Can you work these out from the model? Positions are in its coordinate system, mm. Face numbers are marked on the shaded views. A direction names the side the tool comes from. Give positions to 0.01 mm unless a question says otherwise; leave off trailing zeros. Loops run counter-clockwise (first coordinate to the right, second up) from the corner with the lowest first, then second, coordinate; pieces in that order, holes last. Notation, with made-up numbers: (-14.75, -28.5) - (5.25, -28.5) arc R35 ccw to (5.25, 10.5) - close; hole circle Ø5 at (7, 29.5). An arc over 180 degrees is marked (long way). Answer as a JSON object with one key per item and string values. Group by question number.
Item 1: Which directions (+Z, -Z, +X, -X, +Y, -Y) give clear straight access to the entire face, cutting with the end or side of a thin tool? Please do the marked faces 1, 2 and 3.
Item 2: Thinking about a two-plate mould opening in Y: for the marked faces 4, 5 and 6, which applies, pulls with the +Y half, pulls with the -Y half, needs draft (parallel to the pull), parting line crosses it, or undercut?
Item 3: Please list where these lines run through material, in increasing order: L1, parallel to Y at x = 4, z = 6; L2, parallel to X at y = 6.5, z = 9.75; L3, parallel to Z at x = -2.75, y = -3.5.
Item 4: Will these pins go through, and if not, where does the flat tip stop? pin 1 (1.5 mm diameter, centred on x = -0.5, y = -4.5, fed in from -Z); pin 2 (4.5 mm diameter, centred on x = 0.5, z = 4, fed in from -Y).
Item 5: Suppose I cut it at C-C on x = 0.25. Write out the boundary of the cut face in (y, z).
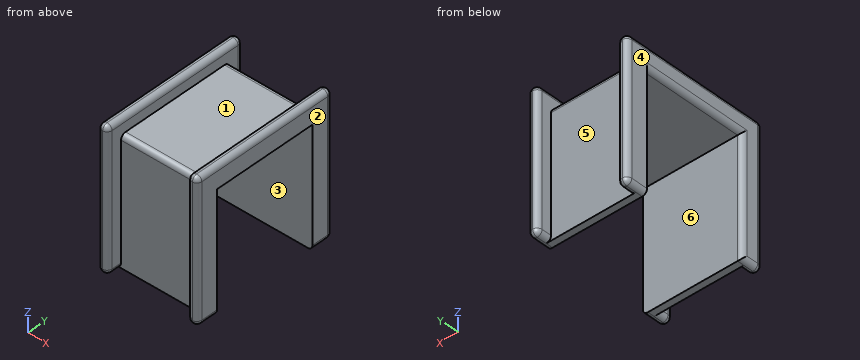
from build123d import *

# Parameters (mm, degrees)
F0_W     = 10.16
F0_H     = 15
F1_DEPTH = 14.28
F2_W     = 8.16
F2_H     = 14.28
F5_DEPTH = 1.5
F3_W     = 8.16
F3_H     = 15
F6_DEPTH = 1.5
F4_W     = 8.16
F4_H     = 14.28
F7_DEPTH = 1.5
F8_W     = 10.6
F8_H     = 12.08
F9_DEPTH = 25
F10_R    = 0.49999


# Not quite as in the source:
# - a fillet or chamfer is up to 0.001 mm smaller than in the source, because OpenCascade refuses the exact size


with BuildPart() as f1:
    # F0 (on Top) → F1 (new body)
    with BuildSketch(Plane.XY):
        Rectangle(F0_W, F0_H)
    extrude(amount=F1_DEPTH)

    # F2 (on face) → F5 (cut)
    with BuildSketch(Plane.XZ.offset(7.5)):
        with Locations((0, 7.14)):
            Rectangle(F2_W, F2_H)
    extrude(amount=-F5_DEPTH, mode=Mode.SUBTRACT)

    # F3 (on face) → F6 (cut)
    with BuildSketch(Plane.XY.offset(14.28)):
        Rectangle(F3_W, F3_H)
    extrude(amount=-F6_DEPTH, mode=Mode.SUBTRACT)

    # F4 (on face) → F7 (cut)
    with BuildSketch(Plane(origin=(0, 7.5, 0), x_dir=(-1, 0, 0), z_dir=(0, 1, 0))):
        with Locations((0, 7.14)):
            Rectangle(F4_W, F4_H)
    extrude(amount=-F7_DEPTH, mode=Mode.SUBTRACT)

    # F8 (on face) → F9 (cut)
    with BuildSketch(Plane.YZ.offset(5.08)):
        with Locations((0, 6.04)):
            Rectangle(F8_W, F8_H)
    extrude(amount=-F9_DEPTH, mode=Mode.SUBTRACT)

    # F10 (radius 0.5 in the source; OpenCascade refuses exactly that, so slightly less here)
    f10_edges = [f1.edges().sort_by_distance(p)[0] for p in [
        (-4.58, -7.5, 14.28),
        (4.58, -7.5, 14.28),
        (-4.08, -7.5, 7.14),
        (-5.08, -7.5, 7.14),
        (-5.08, 0, 14.28),
        (-5.08, 0, 12.08),
        (-5.08, -5.3, 6.04),
        (-5.08, -6.4, 0),
        (-4.58, -7.5, 0),
        (4.58, -7.5, 0),
        (4.08, -7.5, 7.14),
        (5.08, -7.5, 7.14),
        (5.08, 0, 14.28),
        (-4.08, 0, 14.28),
        (4.08, 0, 14.28),
        (5.08, 7.5, 7.14),
        (4.08, 7.5, 7.14),
        (-4.08, 7.5, 7.14),
        (-5.08, 7.5, 7.14),
        (-4.58, 7.5, 14.28),
        (4.58, 7.5, 14.28),
        (4.58, 7.5, 0),
        (-4.58, 7.5, 0),
        (-5.08, 6.4, 0),
        (-4.08, 6.75, 0),
        (4.08, 6.75, 0),
        (5.08, 6.4, 0),
        (5.08, -6.4, 0),
        (-4.08, -6.75, 0),
        (4.08, -6.75, 0),
        (0, -6, 12.78),
        (0, 6, 12.78),
    ]]
    fillet(f10_edges, radius=F10_R)


solid = f1.part
Worked out:
{
 "1": {"face 1": "+Z, +Y, -Y", "face 2": "+Z, -Z, +X, +Y, -Y", "face 3": "-Z, +X, -X"},
 "2": {"face 4": "needs draft", "face 5": "pulls with the +Y half", "face 6": "undercut"},
 "3": {"L1": "y = -6 to -5.3, 5.3 to 6", "L2": "x = -5.08 to -4.08, 4.08 to 5.08", "L3": "z = 12.08 to 12.78"},
 "4": {"pin 1": "stops at z = 12.08", "pin 2": "stops at y = -6"},
 "5": {"outline": "(-6, 0) - (-5.3, 0) - (-5.3, 12.08) - (5.3, 12.08) - (5.3, 0) - (6, 0) - (6, 12.28) arc R0.5 ccw to (5.5, 12.78) - (-5.5, 12.78) arc R0.5 ccw to (-6, 12.28) - close"}
}
